from build123d import *

# Parameters (mm, degrees)
BOX005_W     = 4
BOX005_H     = 2
BOX005_DEPTH = 2
BOX004_W     = 2
BOX004_H     = 4
BOX004_DEPTH = 2
BOX003_W     = 4
BOX003_H     = 2
BOX003_DEPTH = 2
BOX002_W     = 2
BOX002_H     = 4
BOX002_DEPTH = 2
BOX001_W     = 36
BOX001_H     = 36
BOX001_DEPTH = 18
BOX_W        = 40
BOX_H        = 40
BOX_DEPTH    = 20


with BuildPart() as cubo005:
    # Box005 → Box005 (new body)
    with BuildSketch(Plane(origin=(18, 38, 0), x_dir=(1, 0, 0), z_dir=(0, 0, 1))):
        with Locations((2, 1)):
            Rectangle(BOX005_W, BOX005_H)
    extrude(amount=BOX005_DEPTH)


with BuildPart() as cubo004:
    # Box004 → Box004 (new body)
    with BuildSketch(Plane(origin=(38, 18, 0), x_dir=(1, 0, 0), z_dir=(0, 0, 1))):
        with Locations((1, 2)):
            Rectangle(BOX004_W, BOX004_H)
    extrude(amount=BOX004_DEPTH)


with BuildPart() as cubo003:
    # Box003 → Box003 (new body)
    with BuildSketch(Plane(origin=(18, 0, 0), x_dir=(1, 0, 0), z_dir=(0, 0, 1))):
        with Locations((2, 1)):
            Rectangle(BOX003_W, BOX003_H)
    extrude(amount=BOX003_DEPTH)


with BuildPart() as cubo002:
    # Box002 → Box002 (new body)
    with BuildSketch(Plane(origin=(0, 18, 0), x_dir=(1, 0, 0), z_dir=(0, 0, 1))):
        with Locations((1, 2)):
            Rectangle(BOX002_W, BOX002_H)
    extrude(amount=BOX002_DEPTH)


with BuildPart() as cubo001:
    # Box001 → Box001 (new body)
    with BuildSketch(Plane(origin=(2, 2, 0), x_dir=(1, 0, 0), z_dir=(0, 0, 1))):
        with Locations((18, 18)):
            Rectangle(BOX001_W, BOX001_H)
    extrude(amount=BOX001_DEPTH)


with BuildPart() as cut004:
    # Box → Box (new body)
    with BuildSketch(Plane.XY):
        with Locations((20, 20)):
            Rectangle(BOX_W, BOX_H)
    extrude(amount=BOX_DEPTH)

    # Cut: cut Cubo001
    add(cubo001.part, mode=Mode.SUBTRACT)

    # Cut001: cut Cubo002
    add(cubo002.part, mode=Mode.SUBTRACT)

    # Cut002: cut Cubo003
    add(cubo003.part, mode=Mode.SUBTRACT)

    # Cut003: cut Cubo004
    add(cubo004.part, mode=Mode.SUBTRACT)

    # Cut004: cut Cubo005
    add(cubo005.part, mode=Mode.SUBTRACT)


solid = cut004.part
Could you check a few things on this model? Use its own coordinates, in mm. A direction names the side the tool comes from. Coordinates: 2 decimals unless noted, no trailing zeros. Order: outer loops, then holes, each group sorted by start corner. A loop starts at its lowest first (then second) coordinate and runs counter-clockwise, first axis right, second up. Notation, with made-up numbers: (53, 42.5) - (75, 42.5) arc R11 cw to (75, 48.5) - close; hole circle Ø7 at (-13.75, 4). An arc over 180 degrees is marked (long way). Answer in a Markdown table with one row per item. Add a question column.
(1) Will these pins go through, and if not, where does the flat tip stop? pin 1 (1.5 mm diameter, centred on x = 24.5, y = 23.5, fed in from -Z); pin 2 (1.6 mm diameter, centred on x = 20.5, y = 39, fed in from -Z).
(2) I need wall thicknesses on L1, parallel to Y at x = 13, z = 13.5; L2, parallel to Z at x = 13.5, y = 34. Which ranges of each line are inside material? Lowest first, please.
(3) If we section it at A-A, the plane z = 8.25: Please give me the cut outline in (x, y).
(4) On a 3-axis mill with a long thin cutter (end or side, diameter ignored), from which of +Z, -Z, +X, -X, +Y, -Y can I reach the whole of each face in a straight line? I mean faces 1 (the face through (40, 20, 10)), 2 (the face through (5, 1.7, 0)), 3 (the face through (38, 20, 9)), 4 (the face through (20, 39, 2)), 5 (the face through (39, 20, 2)). Say none if no direction works.
(5) If we mould it in two halves opening along Y, with no side actions, what happens to faces 6 (the face through (20, 1, 2)), 7 (the face through (20, 2, 9)), 8 (the face through (20, 0, 10))? For each: released by +Y, released by -Y, zero draft, split by the parting line, or undercut.
(6) If we section it at B-B, the plane x = 10: Please give me the cut outline in (y, z).
Results are:
| question | item | result |
|---|---|---|
| 1 | pin 1 | stops at z = 18 |
| 1 | pin 2 | stops at z = 2 |
| 2 | L1 | y = 0 to 2, 38 to 40 |
| 2 | L2 | z = 18 to 20 |
| 3 | outline | (0, 0) - (40, 0) - (40, 40) - (0, 40) - close; hole (2, 2) - (38, 2) - (38, 38) - (2, 38) - close |
| 4 | face 1 | +Z, -Z, +X, +Y, -Y |
| 4 | face 2 | -Z, +X, -X, +Y, -Y |
| 4 | face 3 | -Z |
| 4 | face 4 | -Z, +Y, -Y |
| 4 | face 5 | -Z, +X, -X |
| 5 | face 6 | zero draft |
| 5 | face 7 | undercut |
| 5 | face 8 | released by -Y |
| 6 | outline | (0, 0) - (2, 0) - (2, 18) - (38, 18) - (38, 0) - (40, 0) - (40, 20) - (0, 20) - close |
